Input: part model. Units: mm. Frame: model coordinates. Face numbers are marked on the shaded views. A direction names the side the tool comes from. Coordinates: 2 decimals unless noted, no trailing zeros. Write each loop counter-clockwise with the first axis right and the second up, starting at its lowest first coordinate (ties: lowest second). Pieces come first, ordered by that corner, then holes. Notation, with made-up numbers: (46.25, 17) -> (75.25, 17) arc R14 ccw to (75.25, 40) -> close; hole circle Ø9 at (23, -4.75). An arc over 180 degrees is marked (long way). Use one line per item in the form item = value. Start each with the question number.
(1) First-contact query: pin 1 (4 mm diameter, centred on x = -7, z = 11, fed in from +Y); pin 2 (6 mm diameter, centred on x = 8.5, z = 19, fed in from -Y); pin 3 (3 mm diameter, centred on x = -4, z = 51.5, fed in from -Y). Flat tips, straight axial feed; report the tip coordinate or a pass-through.
(2) Set-up query: the marked faces 1 and 2. Return all of +Z, -Z, +X, -X, +Y, -Y with unobstructed straight access to the full face (end or side cutting, diameter ignored); none if empty.
(3) Cut plane A-A on y = 0. Return the cut outline in (x, z), plus the area to 3 significant figures.
(4) Ray query, line 1 along Z through (x, y) = (-3.75, -11); line 2 along Y through (x, z) = (-0.25, 6); line 3 along X through (y, z) = (-2.25, 9). Return the intervals inside material, ascending.
(5) Cut plane C-C on z = 10. Return the cut outline in (x, y).
(6) Cut plane D-D on y = 9.25. Return the cut outline in (x, z), plus the area to 3 significant figures.
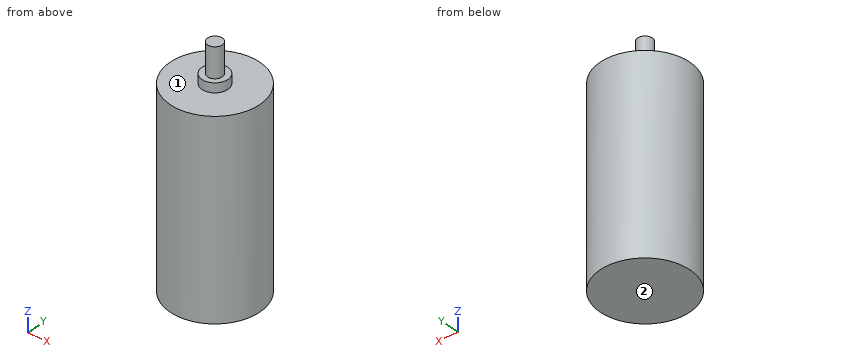
Autodesk Inventor part; units mm, degrees
ref_plane "YZ Plane" through (0, 0, 0) normal (1, 0, 0) x (0, 1, 0)
ref_plane "XZ Plane" through (0, 0, 0) normal (0, 1, 0) x (-1, 0, 0)
ref_plane "XY Plane" through (0, 0, 0) normal (0, 0, 1) x (1, 0, 0)
sketch "Sketch1" plane through (0, 0, 0) normal (0, 0, 1) x (1, 0, 0)
  circle A0 centre (0, 0) radius 12.12
  dimension "d0" = 24.24
extrude "Extrusion1" add sketch "Sketch1" along normal blind 52
sketch "Sketch2" plane through (0, 0, 52) normal (0, 0, 1) x (1, 0, 0)
  circle A0 centre (0, 0) radius 3.5
  dimension "d3" = 7
extrude "Extrusion2" add sketch "Sketch2" along normal blind 2.5
sketch "Sketch3" plane through (0, 0, 54.5) normal (0, 0, 1) x (1, 0, 0)
  circle A0 centre (0, 0) radius 3.5
  circle A1 centre (0, 0) radius 2
  dimension "d6" = 4
extrude "Extrusion3" add sketch "Sketch3" along normal blind 8 contours A1
properties part number "Motorreductor"
Values:
q1.pin_1 = 11.04
q1.pin_2 = -10.8
q1.pin_3 = -11.86
q2.face_1 = +Z
q2.face_2 = -Z, +X, -X, +Y, -Y
q3.outline = (-12.12, 0) -> (12.12, 0) -> (12.12, 52) -> (3.5, 52) -> (3.5, 54.5) -> (2, 54.5) -> (2, 62.5) -> (-2, 62.5) -> (-2, 54.5) -> (-3.5, 54.5) -> (-3.5, 52) -> (-12.12, 52) -> close
q3.area = 1,310 mm2
q4.line_1 = 0 to 52
q4.line_2 = -12.12 to 12.12
q4.line_3 = -11.91 to 11.91
q5.outline = circle Ø24.24 at (0, 0)
q6.outline = (-7.83, 0) -> (7.83, 0) -> (7.83, 52) -> (-7.83, 52) -> close
q6.area = 814 mm2
